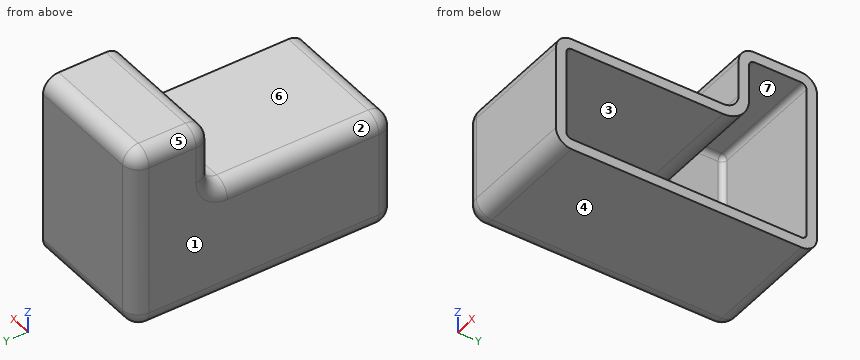
```python
from build123d import *

# Parameters (mm, degrees)
F1_DEPTH = 25
F2_F1_R  = 3
F2_F2_R  = 3
F3_T     = -2


with BuildPart() as f1:
    # F0 (on Right) → F1 (new body)
    with BuildSketch(Plane.YZ):
        Polygon((0, 27.4222218948), (0, 14.4222218948), (-35, 14.4222218948), (-35, -7.5777781052), (15, -7.5777781052), (15, 27.4222218948), align=None)
    extrude(amount=F1_DEPTH)

    # F2: fillet of radius 3 on 11 edges, made by hand

    # F2_f1
    f2_f1_edges = [f1.edges().sort_by_distance(p)[0] for p in [
        (12.5, 0, 14.4222218948),
    ]]
    fillet(f2_f1_edges, radius=F2_F1_R)

    # F2_f2
    f2_f2_edges = [f1.edges().sort_by_distance(p)[0] for p in [
        (0, -10, -7.5777781052),
        (0, -35, 3.4222218948),
        (0, -19, 14.4222218948),
        (0, 7.5, 27.4222218948),
        (0, 15, 9.9222218948),
        (12.5, 15, -7.5777781052),
        (12.5, -35, -7.5777781052),
        (12.5, -35, 14.4222218948),
        (12.5, 0, 27.4222218948),
        (12.5, 15, 27.4222218948),
        (0, -0.8786796564, 15.3009015512),
    ]]
    fillet(f2_f2_edges, radius=F2_F2_R)

    # F3
    f3_openings = [f1.faces().sort_by_distance(p)[0] for p in [
        (25, -7.351061, 6.036173),
    ]]
    offset(amount=F3_T, openings=f3_openings)


solid = f1.part
```
Can you work these out from the model? Positions are in its coordinate system, mm. Face numbers are marked on the shaded views. A direction names the side the tool comes from. Round coordinates to 2 decimals unless told otherwise and drop trailing zeros. Order: outer loops, then holes, each group sorted by start corner. A loop starts at its lowest first (then second) coordinate and runs counter-clockwise, first axis right, second up. Notation, with made-up numbers: (71.5, -29) -> (122.5, -29) arc R16 cw to (122.5, -9) -> close; hole circle Ø4 at (33.5, -2.75). An arc over 180 degrees is marked (long way). Return JSON: item names as keys, results as strings. Group by question number.
1. Which directions (+Z, -Z, +X, -X, +Y, -Y) give clear straight access to the entire face, cutting with the end or side of a thin tool? Please do the marked faces 5, 6 and 7.
2. I need wall thicknesses on line 1 (Z direction, x = 13, y = -14.5); line 2 (Z direction, x = 9.5, y = 4); line 3 (Y direction, x = 13.25, z = -1.5). Which ranges of each line are inside material? Lowest first, please. Write a range as [from, to].
3. If we section it at C-C, the plane z = 6.5: Write out the boundary of the cut face in (x, y), then the cut area to 3 significant figures.
4. If we section it at B-B, the plane x = 18: Write out the boundary of the cut face in (y, z).
5. We'd pull the mould along Z, two halves only. Please class the marked faces 1, 2, 3 and 4: released by +Z, released by -Z, zero draft, split by the parting line, or undercut.
6. Will these pins go through, and if not, where does the flat tip stop? pin 1 (6.5 mm diameter, centred on x = 9, z = 16, fed in from -Y); pin 2 (3.5 mm diameter, centred on x = 17, z = 19.5, fed in from -Y); pin 3 (6.5 mm diameter, centred on x = 15.5, y = -23.5, fed in from +Z).
7. If we section it at A-A, the plane y = 5: Write out the boundary of the cut face in (x, z), then the cut area to 3 significant figures.
Output values:
{
 "1": {"face 5": "+Z, -X, +Y, -Y", "face 6": "+Z, +X, -X, -Y", "face 7": "+X"},
 "2": {"line 1": "[-7.58, -5.58], [12.42, 14.42]", "line 2": "[-7.58, -5.58], [25.42, 27.42]", "line 3": "[-35, -33], [13, 15]"},
 "3": {"outline": "(0, -32) arc R3 ccw to (3, -35) -> (25, -35) -> (25, -33) -> (3, -33) arc R1 cw to (2, -32) -> (2, 12) arc R1 cw to (3, 13) -> (25, 13) -> (25, 15) -> (3, 15) arc R3 ccw to (0, 12) -> close", "area": "189 mm²"},
 "4": {"outline": "(-35, -4.58) arc R3 ccw to (-32, -7.58) -> (12, -7.58) arc R3 ccw to (15, -4.58) -> (15, 24.42) arc R3 ccw to (12, 27.42) -> (3, 27.42) arc R3 ccw to (0, 24.42) -> (0, 17.42) arc R3 cw to (-3, 14.42) -> (-32, 14.42) arc R3 ccw to (-35, 11.42) -> close; hole (-33, -4.58) arc R1 ccw to (-32, -5.58) -> (12, -5.58) arc R1 ccw to (13, -4.58) -> (13, 24.42) arc R1 ccw to (12, 25.42) -> (3, 25.42) arc R1 ccw to (2, 24.42) -> (2, 17.42) arc R5 cw to (-3, 12.42) -> (-32, 12.42) arc R1 ccw to (-33, 11.42) -> close"},
 "5": {"face 1": "zero draft", "face 2": "released by +Z", "face 3": "undercut", "face 4": "released by -Z"},
 "6": {"pin 1": "y = -34.69", "pin 2": "y = 0", "pin 3": "z = 14.42"},
 "7": {"outline": "(0, -4.58) arc R3 ccw to (3, -7.58) -> (25, -7.58) -> (25, -5.58) -> (3, -5.58) arc R1 cw to (2, -4.58) -> (2, 24.42) arc R1 cw to (3, 25.42) -> (25, 25.42) -> (25, 27.42) -> (3, 27.42) arc R3 ccw to (0, 24.42) -> close", "area": "159 mm²"}
}
